from build123d import *

# Parameters (mm, degrees)
SKETCH_1_W                  = 160
SKETCH_1_H                  = 80
EXTRUDE_1_DEPTH             = 4
SKETCH_2_R                  = 3.1
CUT_EXTRUDE_1_DEPTH         = 90.532117142
PATTERN_LINEAR_1_COUNT      = 2
PATTERN_LINEAR_1_PITCH      = 20
PATTERN_LINEAR_1_COUNT_DIR2 = 2
PATTERN_LINEAR_1_PITCH_DIR2 = 130
SKETCH_3_W                  = 110
SKETCH_3_H                  = 36
CUT_EXTRUDE_2_DEPTH         = 90.532117142
SKETCH_4_W                  = 50
SKETCH_4_H                  = 4
EXTRUDE_2_DEPTH             = 10
CHAMFER_1_SIZE              = 4
SKETCH_5_R                  = 9.5
CUT_EXTRUDE_3_DEPTH         = 95.424573073


with BuildPart() as part:
    # 草圖1 → 填料-伸長1 (new body)
    with BuildSketch(Plane.XY):
        Rectangle(SKETCH_1_W, SKETCH_1_H)
    extrude(amount=EXTRUDE_1_DEPTH)

    # 草圖2 → 除料-伸長1 (cut, through all)
    with BuildSketch(Plane.XY.offset(4)):
        with Locations((65, 28)):
            Circle(SKETCH_2_R)
    cut_extrude_1 = extrude(amount=-CUT_EXTRUDE_1_DEPTH, mode=Mode.SUBTRACT)

    # 直線複製排列1: Cut-Extrude 1 2 × 2
    with Locations(*[(-j * PATTERN_LINEAR_1_PITCH_DIR2, -i * PATTERN_LINEAR_1_PITCH, 0) for i in range(PATTERN_LINEAR_1_COUNT) for j in range(PATTERN_LINEAR_1_COUNT_DIR2) if (i, j) != (0, 0)]):
        add(cut_extrude_1, mode=Mode.SUBTRACT)

    # 草圖3 → 除料-伸長2 (cut, through all)
    with BuildSketch(Plane.XY.offset(4)):
        with Locations((25, -22)):
            Rectangle(SKETCH_3_W, SKETCH_3_H)
    extrude(amount=-CUT_EXTRUDE_2_DEPTH, mode=Mode.SUBTRACT)

    # 草圖4 → 填料-伸長2 (add)
    with BuildSketch(Plane.XZ.offset(40)):
        with Locations((-55, 2)):
            Rectangle(SKETCH_4_W, SKETCH_4_H)
    extrude(amount=EXTRUDE_2_DEPTH)

    # 導角1
    chamfer_1_edges = [part.edges().sort_by_distance(p)[0] for p in [
        (80, -4, 2),
        (-30, -4, 2),
        (-80, -50, 2),
        (-30, -50, 2),
        (-80, 40, 2),
        (80, 40, 2),
    ]]
    chamfer(chamfer_1_edges, length=CHAMFER_1_SIZE)

    # 草圖5 → 除料-伸長3 (cut, through all)
    with BuildSketch(Plane.XY.offset(4)):
        with Locations((-55, -30)):
            Circle(SKETCH_5_R)
    extrude(amount=-CUT_EXTRUDE_3_DEPTH, mode=Mode.SUBTRACT)


solid = part.part
Source: CAD feature listing. Evaluate the final solid. Frame: model axes, mm. A direction names the side the tool comes from. Coordinates: 2 decimals unless noted, no trailing zeros. Loops run counter-clockwise (first coordinate to the right, second up) from the corner with the lowest first, then second, coordinate; pieces in that order, holes last. Notation, with made-up numbers: (79, -19) - (106, -19) arc R7 cw to (106, -12) - close; hole circle Ø5 at (45, -37.5). An arc over 180 degrees is marked (long way). Return JSON: item names as keys, results as strings.
Q1. Section B-B, the plane y = 8. Return loops of the section in (x, z), plus the area to 3 significant figures.
Results:
{"outline": "(-80, 0) - (-68.1, 0) - (-68.1, 4) - (-80, 4) - close; (-61.9, 0) - (61.9, 0) - (61.9, 4) - (-61.9, 4) - close; (68.1, 0) - (80, 0) - (80, 4) - (68.1, 4) - close", "area": "590 mm2"}
Q2. Section D-D, the plane y = -37.5. Return loops of the section in (x, z).
Results:
{"outline": "(-80, 0) - (-60.83, 0) - (-60.83, 4) - (-80, 4) - close; (-49.17, 0) - (-30, 0) - (-30, 4) - (-49.17, 4) - close"}
Q3. Contact query for flat-ended pins moving along their axis: P1, Ø2, axis at y = -19, z = 1, coming from the +X side; P2, Ø1.5, axis at x = 37, z = 3, coming from the -Y side; P3, Ø3.5, axis at x = 65, y = 8, coming from the +Z side. Output: stop coordinate, or through.
Results:
{"P1": "x = -30", "P2": "y = -4", "P3": "through"}
Q4. Section A-A, the plane x = -55. Return loops of the section in (y, z).
Results:
{"outline": "(-50, 0) - (-39.5, 0) - (-39.5, 4) - (-50, 4) - close; (-20.5, 0) - (40, 0) - (40, 4) - (-20.5, 4) - close"}
Q5. Material intervals for line 1 along Y through (x, z) = (65, 1.2); line 2 along X through (y, z) = (9, 3.35); line 3 along Y through (x, z) = (-65, 1.5), sorted ascending.
Results:
{"line 1": "-4 to 4.9, 11.1 to 24.9, 31.1 to 40", "line 2": "-80 to -67.93, -62.07 to 62.07, 67.93 to 80", "line 3": "-50 to 4.9, 11.1 to 24.9, 31.1 to 40"}
Q6. Mould query, pull axis X, two halves, no side actions, for faces 1 (the flat face through (-80, -4, 2)), 2 (the flat face through (78, -2, 2)), 3 (the cylindrical face through (-46.224, -33.639, 2.028)), 4 (the flat face through (-1, 40, 2)). Classes: released by +X, released by -X, zero draft, split by the parting line, or undercut.
Results:
{"face 1": "released by -X", "face 2": "released by +X", "face 3": "undercut", "face 4": "zero draft"}
Q7. Section C-C, the plane z = 3.15. Return loops of the section in (x, y).
Results:
{"outline": "(-80, -46) - (-76, -50) - (-34, -50) - (-30, -46) - (-30, -8) - (-26, -4) - (76, -4) - (80, 0) - (80, 36) - (76, 40) - (-76, 40) - (-80, 36) - close; hole circle Ø6.2 at (-65, 8); hole circle Ø6.2 at (-65, 28); hole circle Ø19 at (-55, -30); hole circle Ø6.2 at (65, 8); hole circle Ø6.2 at (65, 28)"}
Q8. Access query for faces 5 (the flat face through (24, -4, 2)), 6 (the flat face through (-78, 38, 2)). Directions: +Z, -Z, +X, -X, +Y, -Y. A direction counts if a zero-diameter tool reaches every point of the face in a straight line with its end or side. Return the directions, or none.
Results:
{"face 5": "+Z, -Z, +X, -Y", "face 6": "+Z, -Z, -X, +Y"}
